Design review of the part built by this model. Coordinates are the model's own, in mm. Face numbers are marked on the shaded views. A direction names the side the tool comes from. Coordinates: 2 decimals unless noted, no trailing zeros. Write each loop counter-clockwise with the first axis right and the second up, starting at its lowest first coordinate (ties: lowest second). Pieces come first, ordered by that corner, then holes. Notation, with made-up numbers: (-27.75, 9) - (27.25, 9) arc R21 ccw to (27.25, 31) - close; hole circle Ø6 at (-16.75, 24.25). An arc over 180 degrees is marked (long way). Use a Markdown table: item, result.
from build123d import *

# Parameters (mm, degrees)
BASE2_DEPTH            = 7.5
MOUNT2_START           = -1.5
MOUNT2_DEPTH           = 3
MOUNT_HOLE2_DEPTH      = 224.418192135
MOUNT_HOLE2_DEPTH_BACK = 224.418192135
SKETCH16_R             = 1.5
SKETCH18_W             = 2.5
SKETCH18_H             = 3.5
SKETCH19_R             = 2
SHAFTHOLE_DEPTH        = 40.784051683
SKETCH20_W             = 20
SKETCH20_H             = 76.405198174
CUT_EXTRUDE10_DEPTH    = 10


with BuildPart() as part:
    # Sketch13 → base2 (new, symmetric)
    with BuildSketch(Plane(origin=(0, 0, 0), x_dir=(1, 0, 0), z_dir=(0, 1, 0))):
        with BuildLine():
            ThreePointArc((-209.761769634, 10), (-208.70564487, 23.279901188), (-206.809628133, 36.46611731))
            Line((-206.809628133, 36.46611731), (-216.657705663, 38.202599087))
            ThreePointArc((-216.657705663, 38.202599087), (-218.670303662, 24.151569236), (-219.772609758, 10))
            Line((-219.772609758, 10), (-209.761769634, 10))
        make_face()
        with BuildLine():
            ThreePointArc((-209.761769634, -10), (-210, 0), (-209.761769634, 10))
            Line((-209.761769634, 10), (-219.772609758, 10))
            ThreePointArc((-219.772609758, 10), (-220, 0), (-219.772609758, -10))
            Line((-219.772609758, -10), (-209.761769634, -10))
        make_face()
        with BuildLine():
            Line((-216.657705663, -38.202599087), (-206.809628133, -36.46611731))
            ThreePointArc((-206.809628133, -36.46611731), (-208.70564487, -23.279901188), (-209.761769634, -10))
            Line((-209.761769634, -10), (-219.772609758, -10))
            ThreePointArc((-219.772609758, -10), (-218.670303662, -24.151569236), (-216.657705663, -38.202599087))
        make_face()
    extrude(amount=BASE2_DEPTH, both=True)

    # Sketch14 → mount2 (cut)
    with BuildSketch(Plane(origin=(0, 0, 0), x_dir=(1, 0, 0), z_dir=(0, 1, 0)).offset(MOUNT2_START)):
        with BuildLine():
            Line((-209.761769634, -10), (-219.772609758, -10))
            ThreePointArc((-219.772609758, -10), (-218.670303662, -24.151569236), (-216.657705663, -38.202599087))
            Line((-216.657705663, -38.202599087), (-206.809628133, -36.46611731))
            ThreePointArc((-206.809628133, -36.46611731), (-208.70564487, -23.279901188), (-209.761769634, -10))
        make_face()
        with BuildLine():
            Line((-209.761769634, 10), (-219.772609758, 10))
            ThreePointArc((-219.772609758, 10), (-218.670303662, 24.151569236), (-216.657705663, 38.202599087))
            Line((-216.657705663, 38.202599087), (-206.809628133, 36.46611731))
            ThreePointArc((-206.809628133, 36.46611731), (-208.70564487, 23.279901188), (-209.761769634, 10))
        make_face()
    extrude(amount=MOUNT2_DEPTH, mode=Mode.SUBTRACT)

    # Sketch16 → mount hole2 (cut, two sides: drawn at the far end of the back side and taken through both)
    with BuildSketch(Plane(origin=(0, 0, 0), x_dir=(1, 0, 0), z_dir=(0, 1, 0)).offset(-MOUNT_HOLE2_DEPTH_BACK)):
        with Locations(Location((-213.160645195, 28.063131327, 0), (0, 0, 270))):
            Circle(SKETCH16_R)
        with Locations(Location((-214.18186009, 18.738484691, 0), (0, 0, 270))):
            Circle(SKETCH16_R)
        with Locations(Location((-214.18186009, -18.738484691, 0), (0, 0, 270))):
            Circle(SKETCH16_R)
        with Locations(Location((-213.160645195, -28.063131327, 0), (0, 0, 270))):
            Circle(SKETCH16_R)
    extrude(amount=MOUNT_HOLE2_DEPTH + MOUNT_HOLE2_DEPTH_BACK, mode=Mode.SUBTRACT)

    # Sketch18 → bearing (revolve, cut)
    with BuildSketch(Plane(origin=(0, 0, 0), x_dir=(1, 0, 0), z_dir=(0, 1, 0)), mode=Mode.PRIVATE) as bearing_sk:
        with Locations((-216.25, 1.75)):
            Rectangle(SKETCH18_W, SKETCH18_H)
    revolve(bearing_sk.sketch.rotate(Axis((-215, 0, 0), (-1, 0, 0)), 180), axis=Axis((-215, 0, 0), (-1, 0, 0)), mode=Mode.SUBTRACT)

    # Sketch19 → shafthole (cut, through all)
    with BuildSketch(Plane(origin=(-215, 0, 0), x_dir=(0, 0, -1), z_dir=(1, 0, 0))):
        Circle(SKETCH19_R)
    extrude(amount=-SHAFTHOLE_DEPTH, mode=Mode.SUBTRACT)

    # Sketch20 → Cut-Extrude10 (cut)
    with BuildSketch(Plane(origin=(0, 0, 0), x_dir=(1, 0, 0), z_dir=(0, 1, 0))):
        with Locations((-210, 0)):
            Rectangle(SKETCH20_W, SKETCH20_H)
    extrude(amount=CUT_EXTRUDE10_DEPTH, mode=Mode.SUBTRACT)


solid = part.part
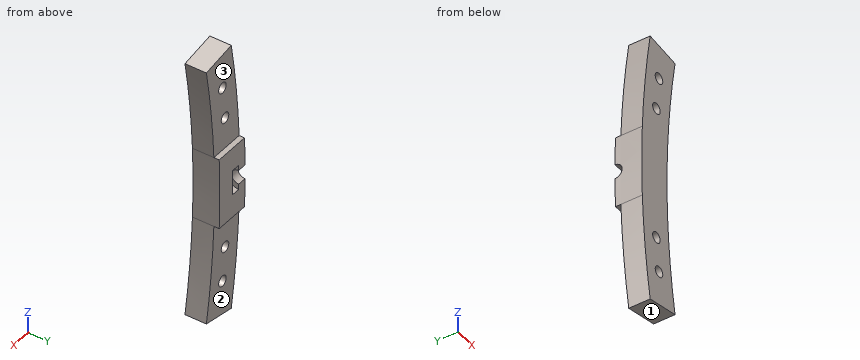
(1) For pin 1 (3 mm diameter, centred on x = -208, y = -3.5, fed in from -Z); pin 2 (1.2 mm diameter, centred on x = -216, y = -1, fed in from -Z); pin 3 (3.5 mm diameter, centred on x = -214.18, z = -18.74, fed in from +Y), all flat-tipped, find the tip position at first contact; note any pin that passes through.
Determined:
| item | result |
|---|---|
| pin 1 | z = -36.94 |
| pin 2 | z = -38.15 |
| pin 3 | y = -1.5 |
(2) Take a section at C-C on y = -4.25. Write out the cut boundary in (x, z), and give its area (3 significant figures).
Determined:
| item | result |
|---|---|
| outline | (-216.66, -38.2) - (-206.81, -36.47) arc R210 cw to (-206.81, 36.47) - (-216.66, 38.2) arc R220 ccw to start; hole circle Ø3 at (-214.18, -18.74); hole circle Ø3 at (-214.18, 18.74); hole circle Ø3 at (-213.16, -28.06); hole circle Ø3 at (-213.16, 28.06) |
| area | 722 mm2 |
(3) Take a section at A-A on z = 0. Write out the cut boundary in (x, y).
Determined:
| item | result |
|---|---|
| outline | (-220, -7.5) - (-210, -7.5) - (-210, 0) - (-215, 0) - (-215, -3.5) - (-217.5, -3.5) - (-217.5, -2) - (-220, -2) - close |
(4) Take a section at B-B on z = 19.5. Write out the cut boundary in (x, y).
Determined:
| item | result |
|---|---|
| outline | (-219.13, -7.5) - (-215.47, -7.5) - (-215.47, -1.5) - (-219.13, -1.5) - close; (-212.89, -7.5) - (-209.09, -7.5) - (-209.09, -1.5) - (-212.89, -1.5) - close |
(5) Machinability: for the marked faces 1, 2 and 3, which of the approach directions +Z, -Z, +X, -X, +Y, -Y give a long, thin tool a straight path to every point of the face, cutting with its end or side? Answer none if there is none.
Determined:
| item | result |
|---|---|
| face 1 | -Z, +X, +Y, -Y |
| face 2 | -Z, +X, -X, +Y |
| face 3 | +Z, +X, -X, +Y |
(6) For L1, parallel to Z at x = -213.75, y = -5.25; L2, parallel to Z at x = -214.75, y = -5; L3, parallel to Y at x = -218, z = -14.5, list the stretches that pass through material, from the lowest coordinate up. Write a range as from..to.
Determined:
| item | result |
|---|---|
| L1 | -37.69..-29.44, -26.68..-20.17, -17.3..17.3, 20.17..26.68, 29.44..37.69 |
| L2 | -37.87..-20.13, -17.35..17.35, 20.13..37.87 |
| L3 | -7.5..-1.5 |
